Model file for the job. Use its own axes, mm. A direction names the side the tool comes from. Round coordinates to 2 decimals unless told otherwise and drop trailing zeros. Order: outer loops, then holes, each group sorted by start corner. A loop starts at its lowest first (then second) coordinate and runs counter-clockwise, first axis right, second up. Notation, with made-up numbers: (10, 11) - (40, 11) arc R29 cw to (40, 33) - close; hole circle Ø11 at (-17, 53.25). An arc over 180 degrees is marked (long way). Use one line per item in the form item = value.
from build123d import *

# Parameters (mm, degrees)
SKETCH1_W                          = 110
SKETCH1_H                          = 35
BOSS_EXTRUDE1_DEPTH                = 6
SKETCH2_W                          = 98
SKETCH2_H                          = 26.5
CUT_EXTRUDE1_DEPTH                 = 6
SKETCH3_W                          = 110
SKETCH3_H                          = 3
CUT_EXTRUDE2_DEPTH                 = 1
CBORE_FOR_M2_5_SHCS1_D             = 2.9
CBORE_FOR_M2_5_SHCS1_CBORE_D       = 4.6
CBORE_FOR_M2_5_SHCS1_CBORE_DEPTH   = 2.5
FILLET1_R                          = 1
TAP_DRILL_FOR_M2_2X0_45_TAP1_D     = 1.75
TAP_DRILL_FOR_M3X0_5_TAP1_D        = 2.5
TAP_DRILL_FOR_M3X0_5_TAP1_DEPTH    = 6
TAP_DRILL_FOR_M3X0_5_TAP1_TIP      = 0.751075774
SKETCH17_W                         = 10
SKETCH17_H                         = 3
SKETCH17_W_2                       = 14
CUT_EXTRUDE3_DEPTH                 = 4
FILLET2_R                          = 0.5
TAP_DRILL_FOR_M3X0_5_TAP2_D        = 2.5
TAP_DRILL_FOR_M3X0_5_TAP2_DEPTH    = 6
TAP_DRILL_FOR_M3X0_5_TAP2_TIP      = 0.751075774
TAP_DRILL_FOR_M2_2X0_45_TAP2_D     = 1.75
TAP_DRILL_FOR_M2_2X0_45_TAP2_DEPTH = 6
TAP_DRILL_FOR_M2_2X0_45_TAP2_TIP   = 0.525753042
TAP_DRILL_FOR_M2_5X0_45_TAP2_D     = 2.05


with BuildPart() as part:
    # Sketch1 → Boss-Extrude1 (new body)
    with BuildSketch(Plane(origin=(0, 0, 0), x_dir=(1, 0, 0), z_dir=(0, 1, 0))):
        with Locations((55, 17.5)):
            Rectangle(SKETCH1_W, SKETCH1_H)
    extrude(amount=BOSS_EXTRUDE1_DEPTH)

    # Sketch2 → Cut-Extrude1 (cut)
    with BuildSketch(Plane(origin=(0, 6, 0), x_dir=(1, 0, 0), z_dir=(0, 1, 0))):
        with Locations((55, 18.25)):
            Rectangle(SKETCH2_W, SKETCH2_H)
    extrude(amount=-CUT_EXTRUDE1_DEPTH, mode=Mode.SUBTRACT)

    # Sketch3 → Cut-Extrude2 (cut)
    with BuildSketch(Plane(origin=(0, 6, 0), x_dir=(1, 0, 0), z_dir=(0, 1, 0))):
        with Locations((55, 2.5)):
            Rectangle(SKETCH3_W, SKETCH3_H)
    extrude(amount=-CUT_EXTRUDE2_DEPTH, mode=Mode.SUBTRACT)

    # CBORE for M2.5 SHCS1 (through all)
    with Locations(Plane(origin=(0, 0, 0), x_dir=(-1, 0, 0), z_dir=(0, -1, 0))):
        with Locations((-100, 2.5), (-10, 2.5)):
            CounterBoreHole(CBORE_FOR_M2_5_SHCS1_D / 2, CBORE_FOR_M2_5_SHCS1_CBORE_D / 2, CBORE_FOR_M2_5_SHCS1_CBORE_DEPTH)

    # Fillet1
    fillet1_edges = [part.edges().sort_by_distance(p)[0] for p in [
        (6, 3, -5),
        (6, 3, -31.5),
        (104, 3, -31.5),
        (104, 3, -5),
    ]]
    fillet(fillet1_edges, radius=FILLET1_R)

    # Tap Drill for M2.2x0.45 Tap1 (through all)
    with Locations(Plane(origin=(0, 0, 0), x_dir=(-1, 0, 0), z_dir=(0, -1, 0))):
        with Locations((-2.5, 2.5), (-107.5, 2.5), (-107.5, 33.25), (-2.5, 33.25)):
            Hole(TAP_DRILL_FOR_M2_2X0_45_TAP1_D / 2)

    # Tap Drill for M3x0.5 Tap1
    with Locations(Plane.XY):
        with Locations((15, 3), (24, 3), (46, 3), (64, 3), (86, 3), (95, 3)):
            Hole(TAP_DRILL_FOR_M3X0_5_TAP1_D / 2, depth=TAP_DRILL_FOR_M3X0_5_TAP1_DEPTH)
            with Locations((0, 0, -(TAP_DRILL_FOR_M3X0_5_TAP1_DEPTH + TAP_DRILL_FOR_M3X0_5_TAP1_TIP / 2))):  # 118° drill point
                Cone(0, TAP_DRILL_FOR_M3X0_5_TAP1_D / 2, TAP_DRILL_FOR_M3X0_5_TAP1_TIP, mode=Mode.SUBTRACT)

    # Sketch17 → Cut-Extrude3 (cut)
    with BuildSketch(Plane.XZ):
        with Locations((55, -2.5)):
            Rectangle(SKETCH17_W, SKETCH17_H)
        with Locations((35.5, -2.5)):
            Rectangle(SKETCH17_W_2, SKETCH17_H)
        with Locations((74.5, -2.5)):
            Rectangle(SKETCH17_W_2, SKETCH17_H)
    extrude(amount=-CUT_EXTRUDE3_DEPTH, mode=Mode.SUBTRACT)

    # Fillet2
    fillet2_edges = [part.edges().sort_by_distance(p)[0] for p in [
        (50, 2, -4),
        (50, 2, -1),
        (60, 2, -1),
        (60, 2, -4),
        (28.5, 2, -4),
        (28.5, 2, -1),
        (42.5, 2, -1),
        (42.5, 2, -4),
        (67.5, 2, -4),
        (67.5, 2, -1),
        (81.5, 2, -1),
        (81.5, 2, -4),
    ]]
    fillet(fillet2_edges, radius=FILLET2_R)

    # Tap Drill for M3x0.5 Tap2
    with Locations(Plane(origin=(0, 0, -35), x_dir=(-1, 0, 0), z_dir=(0, 0, -1))):
        with Locations((-15, 3), (-95, 3)):
            Hole(TAP_DRILL_FOR_M3X0_5_TAP2_D / 2, depth=TAP_DRILL_FOR_M3X0_5_TAP2_DEPTH)
            with Locations((0, 0, -(TAP_DRILL_FOR_M3X0_5_TAP2_DEPTH + TAP_DRILL_FOR_M3X0_5_TAP2_TIP / 2))):  # 118° drill point
                Cone(0, TAP_DRILL_FOR_M3X0_5_TAP2_D / 2, TAP_DRILL_FOR_M3X0_5_TAP2_TIP, mode=Mode.SUBTRACT)

    # Tap Drill for M2.2x0.45 Tap2
    with Locations(Plane(origin=(0, 0, -35), x_dir=(-1, 0, 0), z_dir=(0, 0, -1))):
        with Locations((-24, 4.5), (-46, 4.5), (-64, 4.5), (-86, 4.5)):
            Hole(TAP_DRILL_FOR_M2_2X0_45_TAP2_D / 2, depth=TAP_DRILL_FOR_M2_2X0_45_TAP2_DEPTH)
            with Locations((0, 0, -(TAP_DRILL_FOR_M2_2X0_45_TAP2_DEPTH + TAP_DRILL_FOR_M2_2X0_45_TAP2_TIP / 2))):  # 118° drill point
                Cone(0, TAP_DRILL_FOR_M2_2X0_45_TAP2_D / 2, TAP_DRILL_FOR_M2_2X0_45_TAP2_TIP, mode=Mode.SUBTRACT)

    # Tap Drill for M2.5x0.45 Tap2 (through all)
    with Locations(Plane(origin=(110, 0, 0), x_dir=(0, 0, -1), z_dir=(1, 0, 0))):
        with Locations((6.25, 4.5), (28.75, 4.5)):
            Hole(TAP_DRILL_FOR_M2_5X0_45_TAP2_D / 2)


solid = part.part
(1) Pin check, flat tips, straight feed: pin 1 (2 mm diameter, centred on x = 15, y = 3, fed in from +Z); pin 2 (0.9 mm diameter, centred on x = 73, z = -2.5, fed in from -Y); pin 3 (3.5 mm diameter, centred on x = 99.5, z = -2.5, fed in from -Y); pin 4 (2 mm diameter, centred on x = 46, y = 3, fed in from +Z). Stop position of each tip, or through.
Report:
pin_1 = through
pin_2 = 4
pin_3 = 2.5
pin_4 = -31.5
(2) Slice it at A-A on z = -11. Give the cut face in (x, y), then the cut area to 3 significant figures.
Report:
outline = (0, 0) - (6, 0) - (6, 6) - (0, 6) - close; (104, 0) - (110, 0) - (110, 6) - (104, 6) - close
area = 72.0 mm2
(3) Slice it at D-D on x = 10. Give the cut face in (y, z), then the cut area to 4 significant figures.
Report:
outline = (0, -35) - (6, -35) - (6, -31.5) - (0, -31.5) - close; (0, -5) - (6, -5) - (6, -4) - (5, -4) - (5, -3.95) - (2.5, -3.95) - (2.5, -4.8) - (0, -4.8) - close; (0, -0.2) - (2.5, -0.2) - (2.5, -1.05) - (5, -1.05) - (5, -1) - (6, -1) - (6, 0) - (0, 0) - close
area = 29.25 mm2
(4) Probe probe 1 along Z at (x, y) = (79.5, 3); probe 2 along X at (y, z) = (2.25, -9); probe 3 along Z at (x, y) = (92.5, 0.75). List the from-to ranges inside material, lowest first. Write a range as [from, to].
Report:
probe_1 = [-35, -31.5], [-5, -4], [-1, 0]
probe_2 = [0, 6], [104, 110]
probe_3 = [-35, -31.5], [-5, 0]
(5) Slice it at C-C on x = 35. Give the cut face in (y, z), then the cut area to 3 significant figures.
Report:
outline = (0, -35) - (6, -35) - (6, -31.5) - (0, -31.5) - close; (0, -5) - (6, -5) - (6, -4) - (5, -4) - (5, -1) - (6, -1) - (6, 0) - (0, 0) - (0, -1) - (4, -1) - (4, -4) - (0, -4) - close
area = 36.0 mm2
(6) Pull direction X, two halves, no side cores. Call faces 1 (the face through (64.835, 4.763, -33.226)), 2 (the face through (47, 6, -33)), 3 (the face through (110, 3, -17)): released by +X, released by -X, zero draft, split by the parting line, or undercut.
Report:
face_1 = undercut
face_2 = zero draft
face_3 = released by +X
(7) Slice it at B-B on x = 95. Give the cut face in (y, z), then the cut area to 4 significant figures.
Report:
outline = (0, -35) - (1.75, -35) - (1.75, -31.5) - (0, -31.5) - close; (0, -5) - (1.75, -5) - (1.75, 0) - (0, 0) - close; (4.25, -35) - (6, -35) - (6, -31.5) - (4.25, -31.5) - close; (4.25, -5) - (6, -5) - (6, -4) - (5, -4) - (5, -1) - (6, -1) - (6, 0) - (4.25, 0) - close
area = 26.75 mm2
(8) Tool access for faces 4 (the face through (102.298, 1.232, -2.601)), 5 (the face through (6, 3, -18)), 6 (the face through (106.958, 4.545, -29.774)), 7 (the face through (86.835, 4.763, -33.226)): list every direction of +Z, -Z, +X, -X, +Y, -Y with a clear straight run to the whole face (end or side of a thin tool).
Report:
face_4 = -Y
face_5 = +Y, -Y
face_6 = +X, -X
face_7 = -Z
